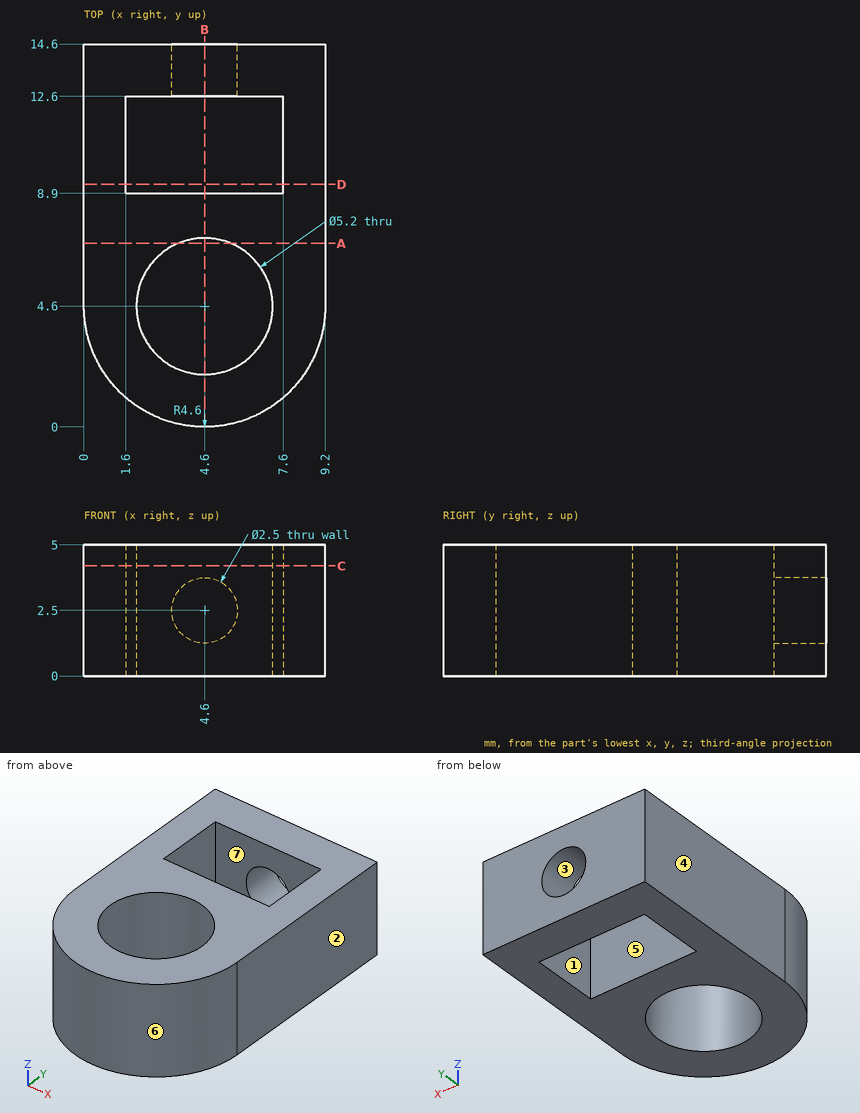
The figure shows three views and two pictorial views of one solid part (mm, origin at its lowest corner). Answer the questions. A direction names the side the tool comes from. Coordinates: 2 decimals unless noted, no trailing zeros. Order: outer loops, then holes, each group sorted by start corner. A loop starts at its lowest first (then second) coordinate and runs counter-clockwise, first axis right, second up. Notation, with made-up numbers: (79.25, 27.25) - (116.25, 27.25) arc R17 cw to (116.25, 32.25) - close; hole circle Ø10 at (58, 53.25). An arc over 180 degrees is marked (long way). Answer as a JSON object with one key per item and string values.
1. The mould has two halves that part along Y. Classify the marked faces 4, 5, 6 and 7: +Y half, -Y half, draft (parallel to the pull), parting line (faces both ways), or undercut.
Output values:
{"face 4": "draft", "face 5": "undercut", "face 6": "-Y half", "face 7": "undercut"}
2. Find section A-A on y = 7. Determine the outline of the cut face in (x, z), plus the area to 3 significant figures.
Output values:
{"outline": "(0, 0) - (3.6, 0) - (3.6, 5) - (0, 5) - close; (5.6, 0) - (9.2, 0) - (9.2, 5) - (5.6, 5) - close", "area": "36.0 mm²"}
3. Consider line 1 (X direction, y = 13.2, z = 2.5); line 2 (Y direction, x = 3, z = 3.85); line 3 (Y direction, x = 6.75, z = 1.65). Determine where each line is inside the solid, lowest interval first.
Output values:
{"line 1": "x = 0 to 3.35, 5.85 to 9.2", "line 2": "y = 0.29 to 2.55, 6.65 to 8.9, 12.6 to 14.6", "line 3": "y = 0.53 to 3.14, 6.06 to 8.9, 12.6 to 14.6"}
4. Each of these flat-tipped pins is pushed along its axis until it touches: P1, Ø4, axis at x = 4.6, y = 4.6, coming from the -Z side; P2, Ø2, axis at x = 4.6, z = 2.5, coming from the +Y side. Where does it stop, or does it pass through?
Output values:
{"P1": "passes through", "P2": "stops at y = 8.9"}
5. A tool of negligible diameter and unlimited length cuts with its end or side. For the marked faces 1, 2 and 3, from which of +Z, -Z, +X, -X, +Y, -Y can it reach the whole face along a straight path? Write none if from no direction.
Output values:
{"face 1": "+Z, -Z", "face 2": "+Z, -Z, +X, +Y, -Y", "face 3": "+Y"}
6. Find section B-B on x = 4.6. Determine the outline of the cut face in (y, z), plus the area to 3 significant figures.
Output values:
{"outline": "(0, 0) - (2, 0) - (2, 5) - (0, 5) - close; (7.2, 0) - (8.9, 0) - (8.9, 5) - (7.2, 5) - close; (12.6, 0) - (14.6, 0) - (14.6, 1.25) - (12.6, 1.25) - close; (12.6, 3.75) - (14.6, 3.75) - (14.6, 5) - (12.6, 5) - close", "area": "23.5 mm²"}
7. Find section D-D on y = 9.25. Determine the outline of the cut face in (x, z), plus the area to 3 significant figures.
Output values:
{"outline": "(0, 0) - (1.6, 0) - (1.6, 5) - (0, 5) - close; (7.6, 0) - (9.2, 0) - (9.2, 5) - (7.6, 5) - close", "area": "16.0 mm²"}
8. Find section C-C on z = 4.2. Determine the outline of the cut face in (x, y).
Output values:
{"outline": "(0, 4.6) arc R4.6 ccw to (9.2, 4.6) - (9.2, 14.6) - (0, 14.6) - close; hole (1.6, 8.9) - (7.6, 8.9) - (7.6, 12.6) - (1.6, 12.6) - close; hole circle Ø5.2 at (4.6, 4.6)"}
